```python
from build123d import *

# Parameters (mm, degrees)
SKETCH1_W           = 35.3
SKETCH1_H           = 24.04
SKETCH1_R           = 1
BOSS_EXTRUDE1_DEPTH = 1.65
SKETCH2_R           = 1
BOSS_EXTRUDE2_DEPTH = 1.65
SKETCH3_R           = 1
BOSS_EXTRUDE3_DEPTH = 1.65
FILLET1_R           = 1
FILLET2_R           = 1
FILLET3_R           = 0.5


with BuildPart() as part:
    # Sketch1 → Boss-Extrude1 (new body)
    with BuildSketch(Plane(origin=(0, 0, 0), x_dir=(1, 0, 0), z_dir=(0, 1, 0))):
        Rectangle(SKETCH1_W, SKETCH1_H)
        with Locations(Location((0, 7.02, 0), (0, 0, 270))):
            Circle(SKETCH1_R, mode=Mode.SUBTRACT)
        with Locations(Location((4.963889604, 4.963889604, 0), (0, 0, 270))):
            Circle(SKETCH1_R, mode=Mode.SUBTRACT)
        with Locations(Location((7.02, 0, 0), (0, 0, 270))):
            Circle(SKETCH1_R, mode=Mode.SUBTRACT)
        with Locations(Location((4.963889604, -4.963889604, 0), (0, 0, 270))):
            Circle(SKETCH1_R, mode=Mode.SUBTRACT)
        with Locations(Location((0, -7.02, 0), (0, 0, 270))):
            Circle(SKETCH1_R, mode=Mode.SUBTRACT)
        with Locations(Location((-4.963889604, -4.963889604, 0), (0, 0, 270))):
            Circle(SKETCH1_R, mode=Mode.SUBTRACT)
        with Locations(Location((-7.02, 0, 0), (0, 0, 270))):
            Circle(SKETCH1_R, mode=Mode.SUBTRACT)
        with Locations(Location((-4.963889604, 4.963889604, 0), (0, 0, 270))):
            Circle(SKETCH1_R, mode=Mode.SUBTRACT)
    extrude(amount=BOSS_EXTRUDE1_DEPTH)

    # Sketch2 → Boss-Extrude2 (add)
    # profile 1 of 2: a face of its own
    with BuildSketch(Plane(origin=(17.65, 0, 0), x_dir=(0, 0, -1), z_dir=(1, 0, 0))):
        Polygon((-7.5, -2.95), (0, -2.95), (0, 0), (-12.02, 0), (-12.02, -11.95), (-7.5, -11.95), align=None)
        with Locations((-10, -8.95)):
            Circle(SKETCH2_R, mode=Mode.SUBTRACT)
    # profile 2 of 2: a face of its own
    with BuildSketch(Plane(origin=(17.65, 0, 0), x_dir=(0, 0, -1), z_dir=(1, 0, 0))):
        Polygon((7.5, -2.95), (7.5, -11.95), (12.02, -11.95), (12.02, 0), (0, 0), (0, -2.95), align=None)
        with Locations((10, -8.95)):
            Circle(SKETCH2_R, mode=Mode.SUBTRACT)
    extrude(amount=-BOSS_EXTRUDE2_DEPTH)

    # Sketch3 → Boss-Extrude3 (add)
    # profile 1 of 2: a face of its own
    with BuildSketch(Plane.ZY.offset(17.65)):
        Polygon((-7.5, -2.95), (0, -2.95), (0, 0), (-12.02, 0), (-12.02, -7.95), (-7.5, -7.95), align=None)
        with Locations((-10, -4.95)):
            Circle(SKETCH3_R, mode=Mode.SUBTRACT)
    # profile 2 of 2: a face of its own
    with BuildSketch(Plane.ZY.offset(17.65)):
        Polygon((7.5, -2.95), (7.5, -7.95), (12.02, -7.95), (12.02, 0), (0, 0), (0, -2.95), align=None)
        with Locations((10, -4.95)):
            Circle(SKETCH3_R, mode=Mode.SUBTRACT)
    extrude(amount=-BOSS_EXTRUDE3_DEPTH)

    # Fillet1
    fillet1_edges = [part.edges().sort_by_distance(p)[0] for p in [
        (17.65, 1.65, 0),
    ]]
    fillet(fillet1_edges, radius=FILLET1_R)

    # Fillet2
    fillet2_edges = [part.edges().sort_by_distance(p)[0] for p in [
        (-17.65, 1.65, 0),
    ]]
    fillet(fillet2_edges, radius=FILLET2_R)

    # Fillet3
    fillet3_edges = [part.edges().sort_by_distance(p)[0] for p in [
        (16.825, -2.95, -7.5),
        (16.825, -2.95, 7.5),
        (16.825, -11.95, 7.5),
        (16.825, -11.95, 12.02),
        (16.825, -11.95, -12.02),
        (16.825, -11.95, -7.5),
        (-16.825, -2.95, 7.5),
        (-16.825, -2.95, -7.5),
        (-16.825, -7.95, -7.5),
        (-16.825, -7.95, -12.02),
        (-16.825, -7.95, 12.02),
        (-16.825, -7.95, 7.5),
    ]]
    fillet(fillet3_edges, radius=FILLET3_R)


solid = part.part
```
Read the model definition and answer for the solid it produces. Units are mm, in the model's axes. A direction names the side the tool comes from. Give positions to 0.01 mm unless a question says otherwise; leave off trailing zeros. Write each loop counter-clockwise with the first axis right and the second up, starting at its lowest first coordinate (ties: lowest second). Pieces come first, ordered by that corner, then holes. Notation, with made-up numbers: M 22.25,44.5 L 75.25,44.5 A12 ccw 75.25,66.5 Z; hole C -4.5,26 d2. An arc over 180 degrees is marked long. Put each result on its own line as item: value. Start each with the question number.
1. The part is cut by section B-B, the plane y = -0.5. Give the vertices of the cut face in (x, z), and give its area (3 significant figures).
2. The part is cut by section C-C, the plane y = -4.95. Give the vertices of the cut face in (x, z).
3. Which of the six approach directions +Z, -Z, +X, -X, +Y, -Y give full straight-line access (tool end or side, diameter ignored) to faces 3 (the flat face through (-17, -2.95, 0)), 4 (the cylindrical face through (16.84, -9.56, -9.21)), 5 (the cylindrical face through (-16.84, -5.56, 9.21)), 6 (the flat face through (-17, -7.95, -10)), 7 (the flat face through (16, -2, 0))?
4. Consider line 1 along X through (y, z) = (-2.5, 1.5); line 2 along X through (y, z) = (1, -4.75); line 3 along Z through (x, y) = (4.5, 0.75). Determine where each line is inside the solid, lowest interval first.
5. For a pull along Z with two mould halves and no side action, classify faces 1 (the cylindrical face through (6.044, 0.813, -0.217)), 2 (the cylindrical face through (-17.349, 1.365, -0.168)) as released by +Z, released by -Z, zero draft, split by the parting line, or undercut.
6. Each of these flat-tipped pins is pushed along its axis until it touches: pin 1 Ø1.2 at (x, z) = (4.96, -4.96) entering from -Y; pin 2 Ø1.8 at (x, z) = (-17, -9) entering from -Y; pin 3 Ø7 at (x, z) = (-6.5, 2) entering from -Y; pin 4 Ø1.3 at (x, z) = (17, 0) entering from -Y. Where does it stop, or does it pass through?
7. The part is cut by section A-A, the plane x = 0. Give the vertices of the cut face in (y, z), and give its area (3 significant figures).
8. The part is cut by section D-D, the plane x = 7.02. Give the vertices of the cut face in (y, z).
Final values:
1. outline: M -17.65,-12.02 L -16,-12.02 L -16,12.02 L -17.65,12.02 Z; M 16,-12.02 L 17.65,-12.02 L 17.65,12.02 L 16,12.02 Z
1. area: 79.3 mm²
2. outline: M -17.65,-12.02 L -16,-12.02 L -16,-11 L -17.65,-11 Z; M -17.65,-9 L -16,-9 L -16,-7.5 L -17.65,-7.5 Z; M -17.65,7.5 L -16,7.5 L -16,9 L -17.65,9 Z; M -17.65,11 L -16,11 L -16,12.02 L -17.65,12.02 Z; M 16,-12.02 L 17.65,-12.02 L 17.65,-7.5 L 16,-7.5 Z; M 16,7.5 L 17.65,7.5 L 17.65,12.02 L 16,12.02 Z
3. face 3: +X, -X, -Y
3. face 4: +X, -X
3. face 5: -X
3. face 6: +Z, -Z, -X, -Y
3. face 7: +Z, -Z, -Y
4. line 1: x = -17.65 to -16, 16 to 17.65
4. line 2: x = -17.59 to -5.94, -3.99 to 3.99, 5.94 to 17.59
4. line 3: z = -12.02 to -5.85, -4.08 to 4.08, 5.85 to 12.02
5. face 1: undercut
5. face 2: zero draft
6. pin 1: passes through
6. pin 2: stops at y = -7.95
6. pin 3: stops at y = 0
6. pin 4: stops at y = -2.95
7. outline: M 0,-12.02 L 1.65,-12.02 L 1.65,-8.02 L 0,-8.02 Z; M 0,-6.02 L 1.65,-6.02 L 1.65,6.02 L 0,6.02 Z; M 0,8.02 L 1.65,8.02 L 1.65,12.02 L 0,12.02 Z
7. area: 33.1 mm²
8. outline: M 0,-12.02 L 1.65,-12.02 L 1.65,-1 L 0,-1 Z; M 0,1 L 1.65,1 L 1.65,12.02 L 0,12.02 Z
